Here's how the part is built. I have some questions about the finished solid (model axes, mm). A direction names the side the tool comes from. Round coordinates to 2 decimals unless told otherwise and drop trailing zeros. Order: outer loops, then holes, each group sorted by start corner. A loop starts at its lowest first (then second) coordinate and runs counter-clockwise, first axis right, second up. Notation, with made-up numbers: (30.25, -11) -> (79.25, -11) arc R18 ccw to (79.25, 20) -> close; hole circle Ø10 at (-5, -28.75). An arc over 180 degrees is marked (long way). Use a Markdown table: item, result. Add a question column.
(1) I want a section at A-A, the plane z = -3.25. Please give me the cut outline in (x, y).
(2) I'm going to push a flat-ended pin straight in: P1, Ø2.5, axis at x = 53.75, y = 0, coming from the +Z side. Where does the tip first touch, or does it pass through?
(3) If I drill on probe 1 along Z at (x, y) = (70, 7.25); probe 2 along Z at (x, y) = (160, 3.5), over which ranges is the centre line in solid material (lowest first)?
(4) Thinking about a two-plate mould opening in Y: for faces 3 (the face through (99, 0, -7.5)), 4 (the face through (99, -6.5, 2)), 5 (the face through (99, -7.5, 2)), which applies, pulls with the +Y half, pulls with the -Y half, needs draft (parallel to the pull), parting line crosses it, or undercut?
(5) On a 3-axis mill with a long thin cutter (end or side, diameter ignored), from which of +Z, -Z, +X, -X, +Y, -Y can I reach the whole of each face in a straight line? I mean faces 1 (the face through (200, 0, 7)), 2 (the face through (99, 0, 6.5)). Say none if no direction works.
(6) I want a section at B-B, the plane x = 134.5. Please give me the cut outline in (y, z).
from build123d import *

# Parameters (mm, degrees)
SKETCH_11_W         = 15
SKETCH_11_H         = 15
SKETCH_11_W_2       = 13
SKETCH_11_H_2       = 13
F_15X15X1_1_DEPTH   = 200
SKETCH_12_R         = 1.45
CUT_EXTRUDE_2_DEPTH = 201.701893364
SKETCH_13_R         = 1.45
CUT_EXTRUDE_3_DEPTH = 201.701893364
SKETCH_14_R         = 1.45
CUT_EXTRUDE_4_DEPTH = 201.701893364
SKETCH_15_R         = 1.45
CUT_EXTRUDE_5_DEPTH = 201.701893364


with BuildPart() as part:
    # 草图11 → 铝管 15X15X1(1) (new body)
    with BuildSketch(Plane(origin=(0, 0, 0), x_dir=(0, 0, -1), z_dir=(1, 0, 0))):
        Rectangle(SKETCH_11_W, SKETCH_11_H)
        Rectangle(SKETCH_11_W_2, SKETCH_11_H_2, mode=Mode.SUBTRACT)
    extrude(amount=F_15X15X1_1_DEPTH)

    # 草图12 → 切除-拉伸2 (cut, through all)
    with BuildSketch(Plane(origin=(0, 7.5, 0), x_dir=(-1, 0, 0), z_dir=(0, -1, 0))):
        with Locations(Location((-100, 0, 0), (0, 0, 90))):
            Circle(SKETCH_12_R)
        with Locations(Location((-190, 0, 0), (0, 0, 90))):
            Circle(SKETCH_12_R)
        with Locations(Location((-10, 0, 0), (0, 0, 90))):
            Circle(SKETCH_12_R)
    extrude(amount=CUT_EXTRUDE_2_DEPTH, mode=Mode.SUBTRACT)

    # 草图13 → 切除-拉伸3 (cut, through all)
    with BuildSketch(Plane.XY.offset(7.5)):
        with Locations((7.5, 0)):
            Circle(SKETCH_13_R)
        with Locations((33.75, 0)):
            Circle(SKETCH_13_R)
        with Locations((53.75, 0)):
            Circle(SKETCH_13_R)
        with Locations(Location((146.25, 0, 0), (0, 0, 180))):
            Circle(SKETCH_13_R)
        with Locations(Location((166.25, 0, 0), (0, 0, 180))):
            Circle(SKETCH_13_R)
        with Locations(Location((192.5, 0, 0), (0, 0, 180))):
            Circle(SKETCH_13_R)
    extrude(amount=-CUT_EXTRUDE_3_DEPTH, mode=Mode.SUBTRACT)

    # 草图14 → 切除-拉伸4 (cut, through all)
    with BuildSketch(Plane.XY.offset(7.5)):
        with Locations((80, 0)):
            Circle(SKETCH_14_R)
        with Locations((120, 0)):
            Circle(SKETCH_14_R)
    extrude(amount=-CUT_EXTRUDE_4_DEPTH, mode=Mode.SUBTRACT)

    # 草图15 → 切除-拉伸5 (cut, through all)
    with BuildSketch(Plane(origin=(0, 7.5, 0), x_dir=(1, 0, 0), z_dir=(0, 1, 0))):
        with Locations(Location((70, 0, 0), (0, 0, 270))):
            Circle(SKETCH_15_R)
        with Locations(Location((130, 0, 0), (0, 0, 270))):
            Circle(SKETCH_15_R)
    extrude(amount=-CUT_EXTRUDE_5_DEPTH, mode=Mode.SUBTRACT)


solid = part.part
Taken from the geometry:
| question | item | result |
|---|---|---|
| 1 | outline | (0, -7.5) -> (200, -7.5) -> (200, -6.5) -> (0, -6.5) -> close; (0, 6.5) -> (200, 6.5) -> (200, 7.5) -> (0, 7.5) -> close |
| 2 | P1 | passes through |
| 3 | probe 1 | z = -7.5 to -1.45, 1.45 to 7.5 |
| 3 | probe 2 | z = -7.5 to -6.5, 6.5 to 7.5 |
| 4 | face 3 | needs draft |
| 4 | face 4 | undercut |
| 4 | face 5 | pulls with the -Y half |
| 5 | face 1 | +Z, -Z, +X, +Y, -Y |
| 5 | face 2 | +X, -X |
| 6 | outline | (-7.5, -7.5) -> (7.5, -7.5) -> (7.5, 7.5) -> (-7.5, 7.5) -> close; hole (-6.5, -6.5) -> (6.5, -6.5) -> (6.5, 6.5) -> (-6.5, 6.5) -> close |
